Autodesk Inventor part; units mm, degrees
ref_plane "YZ Plane" through (0, 0, 0) normal (1, 0, 0) x (0, 1, 0)
ref_plane "XZ Plane" through (0, 0, 0) normal (0, 1, 0) x (-1, 0, 0)
ref_plane "XY Plane" through (0, 0, 0) normal (0, 0, 1) x (1, 0, 0)
sketch "Sketch1" plane through (0, 0, 0) normal (0, 0, 1) x (1, 0, 0)
  line L0 (0, 0) -> (-130, 0)
  line L1 (-130, 0) -> (-130, 62)
  line L2 (-130, 62) -> (0, 62)
  line L3 (0, 62) -> (0, 32.5)
  line L4 (0, 0) -> (20, 0)
  line L5 (20, 0) -> (20, 62)
  line L6 (20, 62) -> (0, 62)
  line L7 (0, 62) -> (0, 0)
  circle A0 centre (0, 30) radius 2.5
  circle A1 centre (14.5, 38.5) radius 2.5
  circle A2 centre (14.5, 51) radius 2.5
  line L8 (14.5, 51) -> (-130, 51)
  line L9 (-115, 0) -> (-95, 0)
  line L10 (-95, 0) -> (-95, -6.4)
  line L11 (-95, -6.4) -> (-115, -6.4)
  line L12 (-115, -6.4) -> (-115, 0)
  line L13 (-65, 0) -> (-45, 0)
  line L14 (-45, 0) -> (-45, -6.4)
  line L15 (-45, -6.4) -> (-65, -6.4)
  line L16 (-65, -6.4) -> (-65, 0)
  line L17 (-15, 0) -> (5, 0)
  line L18 (5, 0) -> (5, -6.4)
  line L19 (5, -6.4) -> (-15, -6.4)
  line L20 (-15, -6.4) -> (-15, 0)
  line L21 (-55, 62) -> (-55, 0)
  line L22 (0, 32.5) -> (0, 27.5)
  line L23 (0, 27.5) -> (0, 0)
  dimension "d0" = 20
  dimension "d1" = 150
  dimension "d2" = 62
  dimension "d3" = 5
  dimension "d4" = 5
  dimension "d5" = 5
  dimension "d6" = 30
  dimension "d7" = 14.5
  dimension "d8" = 8.5
  dimension "d9" = 12.5
  dimension "d10" = 0
  dimension "d11" = 20
  dimension "d12" = 6.4
  dimension "d15" = 50
  dimension "d20" = 75
extrude "Extrusion1" add sketch "Sketch1" along normal blind 5.6 contours L4 L18 L19 L20 L0 | L7 A0 L3 L6 L5 L4 | L0 L21 L8 L3 A0 L7 | L14 L15 L16 L0 | L0 L1 L8 L21 | L8 L21 L2 L3 | L8 L1 L2 L21 | L10 L11 L12 L0
sketch "Sketch3" plane through (0, 0, 5.6) normal (0, 0, 1) x (1, 0, 0)
  circle A0 centre (14.5, 51) radius 2.5
  circle A1 centre (14.5, 38.5) radius 2.5
  circle A2 centre (0, 30) radius 2.5
  line L0 (-115, 0) -> (-115, -6.4)
  line L1 (-115, -6.4) -> (-95, -6.4)
  line L2 (-95, -6.4) -> (-95, 0)
  line L3 (-95, 0) -> (-65, 0)
  line L4 (-65, 0) -> (-65, -6.4)
  line L5 (-65, -6.4) -> (-45, -6.4)
  line L6 (-45, -6.4) -> (-45, 0)
  line L7 (-45, 0) -> (-15, 0)
  line L8 (-15, 0) -> (-15, -6.4)
  line L9 (-15, -6.4) -> (5, -6.4)
  line L10 (5, -6.4) -> (5, 0)
  line L11 (5, 0) -> (20, 0)
  line L12 (20, 0) -> (20, 62)
  line L13 (20, 62) -> (-130, 62)
  line L14 (-130, 62) -> (-130, 0)
  line L15 (-130, 0) -> (-115, 0)
  line L16 (-110, 62) -> (-104.4, 62)
  line L17 (-104.4, 62) -> (-104.4, 32)
  line L18 (-104.4, 32) -> (-110, 32)
  line L19 (-110, 32) -> (-110, 62)
  point P0 (0, 0)
  dimension "d33" = 5.6
  dimension "d34" = 20
  dimension "d35" = 30
sketch "Sketch2" plane through (0, 0, 5.6) normal (0, 0, 1) x (1, 0, 0)
  circle A0 centre (14.5, 51) radius 2.5
  line L0 (20, 62) -> (-130, 62)
  line L1 (-130, 62) -> (-130, 0)
  line L2 (-110, 62) -> (-104.4, 62)
  line L3 (-104.4, 62) -> (-104.4, 51)
  line L4 (-104.4, 51) -> (-110, 51)
  line L5 (-110, 51) -> (-110, 62)
  circle A1 centre (-107.2, 41) radius 1.65
  line L6 (-107.2, 62) -> (-107.2, 51)
  arc A2 (-109.5, 51) -> (-110, 51.5) centre (-110, 51) ccw
  arc A3 (-104.4, 51.5) -> (-104.9, 51) centre (-104.4, 51) ccw
  arc A4 (-104.9, 51) -> (-104.4, 51.5) centre (-104.4, 51) ccw
  arc A5 (-110, 51.5) -> (-109.5, 51) centre (-110, 51) ccw
  point P0 (0, 0)
  dimension "d23" = 5.6
  dimension "d24" = 20
  dimension "d25" = 0
  dimension "d26" = 3.3
  dimension "d27" = 0
  dimension "d28" = 10
  dimension "d31" = 1
  dimension "d32" = 1
equation "\"d1\" = subframe_x"
equation "\"d2\" = subframe_z"
equation "\"d12\" = wood_thickness"
equation "\"d15\" = 0.333333 * subframe_x"
equation "\"d20\" = 0.5 * subframe_x"
equation "\"t_subframe\" = thick_acrylic"
equation "\"d33\" = t_subframe"
equation "\"d23\" = t_subframe"
equation "\"wood_thickness\" = 6.4"
equation "\"m3_diameter\" = 3.15"
equation "\"m5_diameter\" = 5.25"
equation "\"stepper_screw_space\" = 35"
equation "\"stepper_shaft_diameter\" = 5"
equation "\"stepper_body_diameter\" = 28"
equation "\"laser_body_diameter\" = 12"
equation "\"thick_acrylic\" = 5.6"
equation "\"carrier_z\" = 258.6"
equation "\"carrier_z2\" = 283.6"
equation "\"thin_acrylic\" = 3"
equation "\"clear_acrylic\" = 2"
equation "\"linear_bearing_spacing\" = 216"
equation "\"linear_bearing_z\" = 304.8"
equation "\"threaded_rod_z\" = 203.2"
equation "\"motor_spacing\" = 296"
equation "\"tray_boarder\" = 15"
equation "\"bed_clamp_border\" = 15"
equation "\"brass_insert_drill\" = 4"
equation "\"brass_keep_out\" = 8"
equation "\"tape_keep_out\" = 2"
equation "\"tape_thickness\" = 2"
equation "\"crane_x\" = 245.2"
equation "\"crane_z\" = 25"
equation "\"z_min_from_center\" = 72.6"
equation "\"frame_tilt\" = 1deg"
equation "\"printer_z\" = 289"
equation "\"subframe_x\" = 150"
equation "\"subframe_z\" = 62"
properties part number "subframe"
The model under review builds one solid part; all positions refer to its coordinate system, in mm. A direction names the side the tool comes from. Round coordinates to 2 decimals unless told otherwise and drop trailing zeros. Loops run counter-clockwise (first coordinate to the right, second up) from the corner with the lowest first, then second, coordinate; pieces in that order, holes last. Notation, with made-up numbers: (49.5, -13) -> (82.5, -13) arc R32 ccw to (82.5, 20) -> close; hole circle Ø1 at (11, -33). An arc over 180 degrees is marked (long way). Answer as a JSON object with one key per item and string values. Group by question number.
1) We need section D-D on x = -90. Write out the cut boundary in (y, z).
2) For line 1 (Y direction, x = 14.5, z = 1.25); line 2 (X direction, y = 51, z = 1.2); line 3 (Y direction, x = 11, z = 1.4), list the stretches that pass through material, from the lowest coordinate up. Write a range as [from, to].
3) For faces 1 (the face through (-115, -3, 3)), 2 (the face through (12, 0, 3)), 3 (the face through (-30, 0, 3)), list the 3-axis set-ups (+Z, -Z, +X, -X, +Y, -Y) from which the entire face can be reached by the end or side of a thin tool; tool diameter is ignored.
4) We need section A-A on x = 14.5. Write out the cut boundary in (y, z).
5) Mouldability with a two-part tool opening along X and no side actions: class faces 4 (the face through (-55, -6.4, 3)), 5 (the face through (13.96, 53.44, 2.76)), 6 (the face through (-0.33, 27.52, 2.76)), 7 (the face through (-130, 31, 3)) as released by +X, released by -X, zero draft, split by the parting line, or undercut.
6) We need section B-B on z = 3.25. Write out the cut boundary in (x, y).
7) For pin 1 Ø3 at (y, z) = (-2, 4) entering from -X; pin 2 Ø3 at (y, z) = (-3.5, 4) entering from +X, all flat-tipped, find the tip position at first contact; note any pin that passes through.
8) We need section C-C on y = 51. Write out the cut boundary in (x, z), then the cut area to 3 significant figures.
Result set:
{
 "1": {"outline": "(0, 0) -> (62, 0) -> (62, 5.6) -> (0, 5.6) -> close"},
 "2": {"line 1": "[0, 36], [41, 48.5], [53.5, 62]", "line 2": "[-130, 12], [17, 20]", "line 3": "[0, 62]"},
 "3": {"face 1": "+Z, -Z, -X, -Y", "face 2": "+Z, -Z, +X, -Y", "face 3": "+Z, -Z, -Y"},
 "4": {"outline": "(0, 0) -> (36, 0) -> (36, 5.6) -> (0, 5.6) -> close; (41, 0) -> (48.5, 0) -> (48.5, 5.6) -> (41, 5.6) -> close; (53.5, 0) -> (62, 0) -> (62, 5.6) -> (53.5, 5.6) -> close"},
 "5": {"face 4": "zero draft", "face 5": "undercut", "face 6": "undercut", "face 7": "released by -X"},
 "6": {"outline": "(-130, 0) -> (-115, 0) -> (-115, -6.4) -> (-95, -6.4) -> (-95, 0) -> (-65, 0) -> (-65, -6.4) -> (-45, -6.4) -> (-45, 0) -> (-15, 0) -> (-15, -6.4) -> (5, -6.4) -> (5, 0) -> (20, 0) -> (20, 62) -> (-130, 62) -> close; hole circle Ø5 at (0, 30); hole circle Ø5 at (14.5, 38.5); hole circle Ø5 at (14.5, 51)"},
 "7": {"pin 1": "x = -115", "pin 2": "x = 5"},
 "8": {"outline": "(-130, 0) -> (12, 0) -> (12, 5.6) -> (-130, 5.6) -> close; (17, 0) -> (20, 0) -> (20, 5.6) -> (17, 5.6) -> close", "area": "812 mm²"}
}
